from build123d import *

# Parameters (mm, degrees)
F1_DEPTH = 9.5
F2_DEPTH = 11.5
F3_R     = 1.99999
F4_R     = 3


# Not quite as in the source:
# - a fillet or chamfer is up to 0.001 mm smaller than in the source, because OpenCascade refuses the exact size


with BuildPart() as f1:
    # F0 (on Top) → F1 (new body)
    with BuildSketch(Plane.XY):
        with BuildLine():
            Line((6.7996287718, 5.2781800885), (-38.2003712282, 5.2781800885))
            Line((-38.2003712282, 5.2781800885), (-38.2003712282, -29.7218199115))
            Line((-38.2003712282, -29.7218199115), (6.7996287718, -29.7218199115))
            Line((6.7996287718, -29.7218199115), (6.7996287718, -24.2218199115))
            ThreePointArc((6.7996287718, -24.2218199115), (-5.2003712282, -12.2218199115), (6.7996287718, -0.2218199115))
            Line((6.7996287718, -0.2218199115), (6.7996287718, 5.2781800885))
        make_face()
        with BuildLine():
            Line((26.7996287718, 5.2781800885), (6.7996287718, 5.2781800885))
            Line((6.7996287718, 5.2781800885), (6.7996287718, -0.2218199115))
            ThreePointArc((6.7996287718, -0.2218199115), (15.2849101461, -3.7365385373), (18.7996287718, -12.2218199115))
            Line((18.7996287718, -12.2218199115), (26.7996287718, -12.2218199115))
            Line((26.7996287718, -12.2218199115), (26.7996287718, 5.2781800885))
        make_face()
        with BuildLine():
            Line((6.7996287718, -24.2218199115), (6.7996287718, -29.7218199115))
            Line((6.7996287718, -29.7218199115), (26.7996287718, -29.7218199115))
            Line((26.7996287718, -29.7218199115), (26.7996287718, -12.2218199115))
            Line((26.7996287718, -12.2218199115), (18.7996287718, -12.2218199115))
            ThreePointArc((18.7996287718, -12.2218199115), (15.2849101461, -20.7071012858), (6.7996287718, -24.2218199115))
        make_face()
        with BuildLine():
            ThreePointArc((6.7996287718, -24.2218199115), (15.2849101461, -20.7071012858), (18.7996287718, -12.2218199115))
            Line((18.7996287718, -12.2218199115), (16.7996287718, -12.2218199115))
            ThreePointArc((16.7996287718, -12.2218199115), (13.8706965837, -19.2928877234), (6.7996287718, -22.2218199115))
            Line((6.7996287718, -22.2218199115), (6.7996287718, -24.2218199115))
        make_face()
        with BuildLine():
            ThreePointArc((18.7996287718, -12.2218199115), (15.2849101461, -3.7365385373), (6.7996287718, -0.2218199115))
            Line((6.7996287718, -0.2218199115), (6.7996287718, -2.2218199115))
            ThreePointArc((6.7996287718, -2.2218199115), (13.8706965837, -5.1507520997), (16.7996287718, -12.2218199115))
            Line((16.7996287718, -12.2218199115), (18.7996287718, -12.2218199115))
        make_face()
        with BuildLine():
            Line((6.7996287718, -2.2218199115), (6.7996287718, -0.2218199115))
            ThreePointArc((6.7996287718, -0.2218199115), (-5.2003712282, -12.2218199115), (6.7996287718, -24.2218199115))
            Line((6.7996287718, -24.2218199115), (6.7996287718, -22.2218199115))
            ThreePointArc((6.7996287718, -22.2218199115), (-3.2003712282, -12.2218199115), (6.7996287718, -2.2218199115))
        make_face()
        with BuildLine():
            Line((6.7996287718, -22.2218199115), (6.7996287718, -2.2218199115))
            ThreePointArc((6.7996287718, -2.2218199115), (-3.2003712282, -12.2218199115), (6.7996287718, -22.2218199115))
        make_face()
        with BuildLine():
            ThreePointArc((16.7996287718, -12.2218199115), (13.8706965837, -5.1507520997), (6.7996287718, -2.2218199115))
            Line((6.7996287718, -2.2218199115), (6.7996287718, -22.2218199115))
            ThreePointArc((6.7996287718, -22.2218199115), (13.8706965837, -19.2928877234), (16.7996287718, -12.2218199115))
        make_face()
    extrude(amount=F1_DEPTH)

    # F0 (on Top) → F2 (join)
    with BuildSketch(Plane.XY):
        with BuildLine():
            ThreePointArc((6.7996287718, -24.2218199115), (15.2849101461, -20.7071012858), (18.7996287718, -12.2218199115))
            Line((18.7996287718, -12.2218199115), (16.7996287718, -12.2218199115))
            ThreePointArc((16.7996287718, -12.2218199115), (13.8706965837, -19.2928877234), (6.7996287718, -22.2218199115))
            Line((6.7996287718, -22.2218199115), (6.7996287718, -24.2218199115))
        make_face()
        with BuildLine():
            ThreePointArc((18.7996287718, -12.2218199115), (15.2849101461, -3.7365385373), (6.7996287718, -0.2218199115))
            Line((6.7996287718, -0.2218199115), (6.7996287718, -2.2218199115))
            ThreePointArc((6.7996287718, -2.2218199115), (13.8706965837, -5.1507520997), (16.7996287718, -12.2218199115))
            Line((16.7996287718, -12.2218199115), (18.7996287718, -12.2218199115))
        make_face()
        with BuildLine():
            Line((6.7996287718, -2.2218199115), (6.7996287718, -0.2218199115))
            ThreePointArc((6.7996287718, -0.2218199115), (-5.2003712282, -12.2218199115), (6.7996287718, -24.2218199115))
            Line((6.7996287718, -24.2218199115), (6.7996287718, -22.2218199115))
            ThreePointArc((6.7996287718, -22.2218199115), (-3.2003712282, -12.2218199115), (6.7996287718, -2.2218199115))
        make_face()
    extrude(amount=F2_DEPTH)

    # F3 (radius 2 in the source; OpenCascade refuses exactly that, so slightly less here)
    f3_edges = [f1.edges().sort_by_distance(p)[0] for p in [
        (6.799629, -24.22182, 11.5),
    ]]
    fillet(f3_edges, radius=F3_R)

    # F4
    f4_edges = [f1.edges().sort_by_distance(p)[0] for p in [
        (-5.700371, -29.72182, 9.5),
        (26.799629, -12.22182, 9.5),
        (26.799629, -29.72182, 4.75),
        (-38.200371, -29.72182, 4.75),
        (-38.200371, -12.22182, 9.5),
        (-38.200371, 5.27818, 4.75),
        (26.799629, 5.27818, 4.75),
        (-5.700371, 5.27818, 9.5),
    ]]
    fillet(f4_edges, radius=F4_R)


solid = f1.part
For this review, take the finished solid that the model builds, in its own axes (mm). Give positions to 0.01 mm unless a question says otherwise; leave off trailing zeros. Loops run counter-clockwise (first coordinate to the right, second up) from the corner with the lowest first, then second, coordinate; pieces in that order, holes last.
Item 1: Take a section at B-B, the plane x = -10. State the section outline as (y, z) points.
Item 2: Insertion check: pin 1 (4 mm diameter, centred on y = 1.5, z = 9.5, fed in from +X); pin 2 (5 mm diameter, centred on x = -17, z = 9.5, fed in from +Y); pin 3 (5 mm diameter, centred on x = 10, y = -11.5, fed in from +Z). Each pin has a flat end and moves straight along its axis. Give the tip position at first contact, or say it passes through.
Item 3: Draft analysis for pull direction Y (two halves, no side actions). For faces 1 (the cylindrical face through (-6.11, 4.38, 8.64)), 2 (the flat face through (7, -12, 9.5)), 3 (the flat face through (26.8, -12, 3)), state which applies: +Y half, -Y half, draft (parallel to the pull), parting line (faces both ways), or undercut.
Item 4: Take a section at A-A, the plane z = 7.5. State the section outline as (x, y) points, and give its area (3 significant figures).
Item 5: Take a section at C-C, the plane y = 3.5. State the section outline as (x, z) points, and give its area (3 significant figures).
Item 6: Take a section at D-D, the plane z = 10.75. State the section outline as (x, y) points, and give its area (3 significant figures).
Item 7: For line 1 along Z through (x, y) = (-28, -13); line 2 along X through (y, z) = (-19.5, 10.25); line 3 along X through (y, z) = (-8, 6.75), list the stretches that pass through material, from the lowest coordinate up.
Calculated:
1. outline: (-29.72, 0) - (5.28, 0) - (5.28, 6.5) arc R3 ccw to (2.28, 9.5) - (-26.72, 9.5) arc R3 ccw to (-29.72, 6.5) - close
2. pin 1: stops at x = 26.63
2. pin 2: stops at y = 5.24
2. pin 3: stops at z = 9.5
3. face 1: +Y half
3. face 2: undercut
3. face 3: draft
4. outline: (-38.03, -26.72) arc R2.83 ccw to (-35.2, -29.55) - (23.8, -29.55) arc R2.83 ccw to (26.63, -26.72) - (26.63, 2.28) arc R2.83 ccw to (23.8, 5.11) - (-35.2, 5.11) arc R2.83 ccw to (-38.03, 2.28) - close
4. area: 2,230 mm2
5. outline: (-37.94, 0) - (26.54, 0) - (26.54, 6.5) arc R2.74 ccw to (23.8, 9.24) - (-35.2, 9.24) arc R2.74 ccw to (-37.94, 6.5) - close
5. area: 593 mm2
6. outline: circle Ø23.12 at (6.8, -12.22); hole circle Ø20 at (6.8, -12.22)
6. area: 106 mm2
7. line 1: z = 0 to 9.5
7. line 2: x = -2.56 to -0.06, 13.66 to 16.16
7. line 3: x = -38.19 to 26.79
